```python
from build123d import *

# Parameters (mm, degrees)
SKETCH1_R           = 2.85
BOSS_EXTRUDE1_DEPTH = 60
SKETCH2_R           = 9.141
BOSS_EXTRUDE2_DEPTH = 2
BOSS_EXTRUDE3_DEPTH = 32.5
SKETCH4_W           = 2
SKETCH4_H           = 2
CUT_EXTRUDE1_DEPTH  = 15
SKETCH5_R           = 3.5
BOSS_EXTRUDE5_DEPTH = 1


with BuildPart() as part:
    # Sketch1 → Boss-Extrude1 (new body)
    with BuildSketch(Plane.YZ):
        with Locations(Location((0, 0, 0), (0, 0, 270))):
            Circle(SKETCH1_R)
    extrude(amount=BOSS_EXTRUDE1_DEPTH)

    # Sketch2 → Boss-Extrude2 (add)
    with BuildSketch(Plane(origin=(0, 0, 0), x_dir=(0, -1, 0), z_dir=(-1, 0, 0))):
        with Locations(Location((0, 0, 0), (0, 0, 90))):
            Circle(SKETCH2_R)
    extrude(amount=BOSS_EXTRUDE2_DEPTH)

    # Sketch3 → Boss-Extrude3 (add)
    with BuildSketch(Plane.YZ):
        Polygon((3.665, 6.34796621), (-3.665, 6.34796621), (-7.33, 0), (-3.665, -6.34796621), (3.665, -6.34796621), (7.33, 0), align=None)
    extrude(amount=BOSS_EXTRUDE3_DEPTH)

    # Sketch4 → Cut-Extrude1 (cut)
    with BuildSketch(Plane.YZ.offset(60)):
        with Locations((1.85, 0)):
            Rectangle(SKETCH4_W, SKETCH4_H)
    extrude(amount=-CUT_EXTRUDE1_DEPTH, mode=Mode.SUBTRACT)

    # Sketch5 → Boss-Extrude5 (add)
    with BuildSketch(Plane.YZ.offset(32.5)):
        with Locations(Location((0, 0, 0), (0, 0, 270))):
            Circle(SKETCH5_R)
    extrude(amount=BOSS_EXTRUDE5_DEPTH)


solid = part.part
```
Can you work these out from the model? Positions are in its coordinate system, mm. A direction names the side the tool comes from. Coordinates: 2 decimals unless noted, no trailing zeros. Loops run counter-clockwise (first coordinate to the right, second up) from the corner with the lowest first, then second, coordinate; pieces in that order, holes last. Notation, with made-up numbers: M -4.5,5.25 L 3.5,5.25 A27 ccw 3.5,21.25 Z; hole C 26.5,42.5 d9. An arc over 180 degrees is marked long. Put each result on its own line as item: value. Start each with the question number.
(1) Imagine slicing it at B-B on z = -4.25. List the corners of the cut face in (x, y) for me, and give its area (3 significant figures).
(2) Imagine slicing it at C-C on x = 3. List the corners of the cut face in (y, z) for me (3 decimals), and give its area (3 significant figures).
(3) Which directions (+Z, -Z, +X, -X, +Y, -Y) give clear straight access to the entire face, cutting with the end or side of a thin tool? Please do faces 4 (the face through (46.56, -2.78, 0.62)), 5 (the face through (16.02, 5.47, -3.22)), 6 (the face through (16.02, -5.47, 3.22)), 7 (the face through (16.022, 5.523, 3.13)).
(4) Imagine slicing it at A-A on y = 0. List the corners of the cut face in (x, z) for me, and give its area (3 significant figures).
(5) I need wall thicknesses on probe 1 along X at (y, z) = (-1, -8.5); probe 2 along Z at (x, y) = (37.5, 0.25); probe 3 along X at (y, z) = (-6, 1.25). Which ranges of each line are inside material? Lowest first, please.
(6) Will these pins go through, and if not, where does the flat tip stop? pin 1 Ø1 at (x, y) = (22.5, -2.5) entering from +Z; pin 2 Ø6 at (x, z) = (47.5, 0) entering from +Y; pin 3 Ø2 at (x, y) = (24.5, 4.5) entering from -Z.
(7) Imagine slicing it at D-D on z = 5.5. List the corners of the cut face in (x, y) for me.
(8) We'd pull the mould along Z, two halves only. Please class faces 1 (the face through (60, 0, 0)), 2 (the face through (53, 0.85, 0)), 3 (the face through (16, 0, 6.348)): +Z half, -Z half, draft (parallel to the pull), parting line (faces both ways), or undercut.
Worked answers:
1. outline: M -2,-8.09 L 0,-8.09 L 0,-4.88 L 32.5,-4.88 L 32.5,4.88 L 0,4.88 L 0,8.09 L -2,8.09 Z
1. area: 349 mm2
2. outline: M -7.33,0 L -3.665,-6.348 L 3.665,-6.348 L 7.33,0 L 3.665,6.348 L -3.665,6.348 Z
2. area: 140 mm2
3. face 4: +X
3. face 5: -Z, +X, +Y
3. face 6: +Z, +X, -Y
3. face 7: +Z, +X, +Y
4. outline: M -2,-9.14 L 0,-9.14 L 0,-6.35 L 32.5,-6.35 L 32.5,-3.5 L 33.5,-3.5 L 33.5,-2.85 L 60,-2.85 L 60,2.85 L 33.5,2.85 L 33.5,3.5 L 32.5,3.5 L 32.5,6.35 L 0,6.35 L 0,9.14 L -2,9.14 Z
4. area: 607 mm2
5. probe 1: x = -2 to 0
5. probe 2: z = -2.84 to 2.84
5. probe 3: x = -2 to 32.5
6. pin 1: stops at z = 6.35
6. pin 2: stops at y = 2.85
6. pin 3: stops at z = -6.35
7. outline: M -2,-7.3 L 0,-7.3 L 0,-4.15 L 32.5,-4.15 L 32.5,4.15 L 0,4.15 L 0,7.3 L -2,7.3 Z
8. face 1: draft
8. face 2: undercut
8. face 3: +Z half
